```python
from build123d import *

# Parameters (mm, degrees)
SKETCH_1_R      = 2.55
EXTRUDE_1_DEPTH = 6


with BuildPart() as part:
    # Эскиз1 → Бобышка-Вытянуть1 (new body)
    with BuildSketch(Plane.XY):
        with BuildLine():
            Line((10, -4), (5, -4))
            Line((5, -4), (-10, -4))
            ThreePointArc((-10, -4), (-14, 0), (-10, 4))
            Line((-10, 4), (10, 4))
            ThreePointArc((10, 4), (14, 0), (10, -4))
        make_face()
        with Locations((10, 0)):
            Circle(SKETCH_1_R, mode=Mode.SUBTRACT)
        with Locations((-10, 0)):
            Circle(SKETCH_1_R, mode=Mode.SUBTRACT)
    extrude(amount=EXTRUDE_1_DEPTH)


solid = part.part
```
Source: CAD feature listing. Evaluate the final solid. Frame: model axes, mm. Coordinates: 2 decimals unless noted, no trailing zeros. Order: outer loops, then holes, each group sorted by start corner. A loop starts at its lowest first (then second) coordinate and runs counter-clockwise, first axis right, second up. Notation, with made-up numbers: M 14,89 L 19,89 A21 cw 19,97 Z; hole C 81.25,21 d4. An arc over 180 degrees is marked long. Write each question's results on one line, items separated by ' | '. Start each with the question number.
1) Section query A-A (y = 0). Return the cut outline in (x, z), plus the area to 3 significant figures.
2) Section query C-C (y = 1.25). Return the cut outline in (x, z), plus the area to 3 significant figures.
3) Line query: line 1 (Y direction, x = 10, z = 3.9); line 2 (X direction, y = -0.25, z = 2.4); line 3 (X direction, y = -2.25, z = 1.05). Output: solid intervals per line, ascending. Write a range as from..to.
4) Section query D-D (y = -3.5). Return the cut outline in (x, z).
5) Section query B-B (z = 0.5). Return the cut outline in (x, y).
6) Contact query for flat-ended pins moving along their axis: pin 1 Ø1.5 at (y, z) = (1, 3.5) entering from +X; pin 2 Ø3 at (y, z) = (2.5, 4) entering from +X; pin 3 Ø3 at (x, y) = (-10, 0) entering from -Z. Output: stop coordinate, or through.
7) Draft query along X for faces 1 (the face through (-14, 0, 3)), 2 (the face through (0, 4, 3)), 3 (the face through (12.43, 0.77, 2.96)). Return one class per face: released by +X, released by -X, zero draft, split by the parting line, or undercut.
Answers:
1) outline: M -14,0 L -12.55,0 L -12.55,6 L -14,6 Z; M -7.45,0 L 7.45,0 L 7.45,6 L -7.45,6 Z; M 12.55,0 L 14,0 L 14,6 L 12.55,6 Z | area: 107 mm^2
2) outline: M -13.8,0 L -12.22,0 L -12.22,6 L -13.8,6 Z; M -7.78,0 L 7.78,0 L 7.78,6 L -7.78,6 Z; M 12.22,0 L 13.8,0 L 13.8,6 L 12.22,6 Z | area: 112 mm^2
3) line 1: y = -4..-2.55, 2.55..4 | line 2: x = -13.99..-12.54, -7.46..7.46, 12.54..13.99 | line 3: x = -13.31..-11.2, -8.8..8.8, 11.2..13.31
4) outline: M -11.94,0 L 11.94,0 L 11.94,6 L -11.94,6 Z
5) outline: M -10,-4 L 10,-4 A4 ccw 10,4 L -10,4 A4 ccw Z; hole C -10,0 d5.1; hole C 10,0 d5.1
6) pin 1: stops at x = 13.99 | pin 2: stops at x = 13.87 | pin 3: passes through
7) face 1: released by -X | face 2: zero draft | face 3: undercut
